Design review of the part built by this model. Coordinates are the model's own, in mm. Face numbers are marked on the shaded views. Round coordinates to 2 decimals unless told otherwise and drop trailing zeros. Write each loop counter-clockwise with the first axis right and the second up, starting at its lowest first coordinate (ties: lowest second). Pieces come first, ordered by that corner, then holes. Notation, with made-up numbers: M 60.5,18.5 L 64.5,18.5 A16 cw 64.5,42.5 Z; hole C -32.5,70.5 d2. An arc over 180 degrees is marked long. Use CSV: the item, a comma, the result in double quotes.
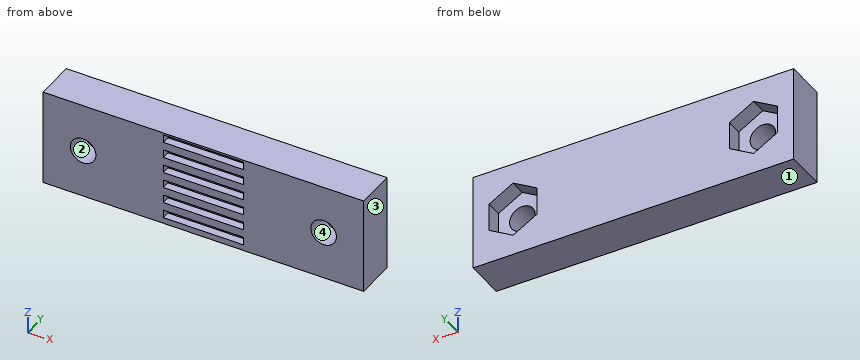
from build123d import *

# Parameters (mm, degrees)
SKETCH1_W           = 40
SKETCH1_H           = 12
BOSS_EXTRUDE1_DEPTH = 5
SKETCH2_R           = 1.6
CUT_EXTRUDE2_DEPTH  = 22.470910554
TEETH_DEPTH         = 5
TEETH_DEPTH_BACK    = 5
TEETH_START         = -20
SKETCH3_W           = 1
SKETCH3_H           = 1
CUT_EXTRUDE4_DEPTH  = 2


with BuildPart() as part:
    # Sketch1 → Boss-Extrude1 (new body)
    with BuildSketch(Plane(origin=(0, 0, 0), x_dir=(1, 0, 0), z_dir=(0, 1, 0))):
        Rectangle(SKETCH1_W, SKETCH1_H)
    extrude(amount=BOSS_EXTRUDE1_DEPTH)

    # Sketch2 → Cut-Extrude2 (cut, through all)
    with BuildSketch(Plane(origin=(0, 5, 0), x_dir=(1, 0, 0), z_dir=(0, 1, 0))):
        with Locations(Location((15, 0, 0), (0, 0, 270))):
            Circle(SKETCH2_R)
        with Locations(Location((-15, 0, 0), (0, 0, 90))):
            Circle(SKETCH2_R)
    extrude(amount=-CUT_EXTRUDE2_DEPTH, mode=Mode.SUBTRACT)

    # Sketch3 → Teeth (cut, two sides: drawn at the far end of the back side and taken through both)
    with BuildSketch(Plane.ZY.offset(20).offset(TEETH_START - TEETH_DEPTH_BACK)):
        with Locations((-4.75, 0.5)):
            Rectangle(SKETCH3_W, SKETCH3_H)
        with Locations((-2.75, 0.5)):
            Rectangle(SKETCH3_W, SKETCH3_H)
        with Locations((-0.75, 0.5)):
            Rectangle(SKETCH3_W, SKETCH3_H)
        with Locations((1.25, 0.5)):
            Rectangle(SKETCH3_W, SKETCH3_H)
        with Locations((3.25, 0.5)):
            Rectangle(SKETCH3_W, SKETCH3_H)
        with Locations((5.25, 0.5)):
            Rectangle(SKETCH3_W, SKETCH3_H)
        with Locations((7.25, 0.5)):
            Rectangle(SKETCH3_W, SKETCH3_H)
        with Locations((9.25, 0.5)):
            Rectangle(SKETCH3_W, SKETCH3_H)
    extrude(amount=TEETH_DEPTH + TEETH_DEPTH_BACK, mode=Mode.SUBTRACT)

    # Sketch4 → Cut-Extrude4 (cut)
    with BuildSketch(Plane(origin=(0, 5, 0), x_dir=(1, 0, 0), z_dir=(0, 1, 0))):
        Polygon((-15, 3.464101615), (-18, 1.732050808), (-18, -1.732050808), (-15, -3.464101615), (-12, -1.732050808), (-12, 1.732050808), align=None)
        Polygon((12, 1.732050808), (15, 3.464101615), (18, 1.732050808), (18, -1.732050808), (15, -3.464101615), (12, -1.732050808), align=None)
    extrude(amount=-CUT_EXTRUDE4_DEPTH, mode=Mode.SUBTRACT)


solid = part.part
1) Wall thickness on line 1 along X through (y, z) = (2.2, 0); line 2 along X through (y, z) = (0.55, 5.25); line 3 along X through (y, z) = (3.7, 3.25): over which ranges is each line inside the solid? List them lowest first. Write a range as [from, to].
Answers:
line 1,"[-20, -16.6], [-13.4, 13.4], [16.6, 20]"
line 2,"[-20, -5], [5, 20]"
line 3,"[-20, -15.37], [-14.63, 14.63], [15.37, 20]"
2) Add section A-A on y = 0.55. Give the number of separate pieces and of enclosed holes in the cut face, then the cut area to 3 significant figures.
Answers:
separate pieces,"1"
enclosed holes,"8"
area,"404 mm²"
3) For pin 1 Ø3 at (x, z) = (-14.5, -1) entering from +Y, flat-tipped, find the tip position at first contact; note if it passes through.
Answers:
pin 1,"y = 3"
4) Add section C-C on y = 3.45. Write out the cut boundary in (x, z).
Answers:
outline,"M -20,-6 L 20,-6 L 20,6 L -20,6 Z; hole M -18,-1.73 L -15,-3.46 L -12,-1.73 L -12,1.73 L -15,3.46 L -18,1.73 Z; hole M 12,-1.73 L 15,-3.46 L 18,-1.73 L 18,1.73 L 15,3.46 L 12,1.73 Z"
5) The part is to be moulded in two halves that separate along X. For the marked faces 1, 2, 3 and 4, say which applies: released by +X, released by -X, zero draft, split by the parting line, or undercut.
Answers:
face 1,"zero draft"
face 2,"undercut"
face 3,"released by +X"
face 4,"undercut"
6) Add section B-B on x = -4.5. Write out the cut boundary in (y, z), then the cut area to 3 significant figures.
Answers:
outline,"M 0,-6 L 5,-6 L 5,6 L 0,6 L 0,5.75 L 1,5.75 L 1,4.75 L 0,4.75 L 0,3.75 L 1,3.75 L 1,2.75 L 0,2.75 L 0,1.75 L 1,1.75 L 1,0.75 L 0,0.75 L 0,-0.25 L 1,-0.25 L 1,-1.25 L 0,-1.25 L 0,-2.25 L 1,-2.25 L 1,-3.25 L 0,-3.25 L 0,-4.25 L 1,-4.25 L 1,-5.25 L 0,-5.25 Z"
area,"54.0 mm²"
